Drawing for the job (mm, zero at the part's lowest x, y, z). A direction names the side the tool comes from. Coordinates: 2 decimals unless noted, no trailing zeros. Write each loop counter-clockwise with the first axis right and the second up, starting at its lowest first coordinate (ties: lowest second). Pieces come first, ordered by that corner, then holes. Notation, with made-up numbers: M 40.5,68.25 L 70.5,68.25 A10 cw 70.5,86.25 Z; hole C 5,58.5 d2. An arc over 180 degrees is marked long. Put each result on its own line as item: value. Start each with the question number.
Q1. Cut at A-A (z = 21.5). Write the cut outline in (x, y), then the cut area to 3 significant figures.
Q2. Drill centre lines: line 1 along X through (y, z) = (1.6, 21.25); line 2 along Z through (x, y) = (38.5, 2.2); line 3 along X through (y, z) = (1.25, 5.25). Where is each one in solid material? Low to high.
Q3. Which spindle directions (+Z, -Z, +X, -X, +Y, -Y) get a long thin tool onto all of the face, cutting with end or side? Do the marked faces 1, 2 and 3. Say none if no direction does.
Q4. Drop flat-ended pins along their axis: pin 1 (1.2 mm diameter, centred on y = 1.5, z = 5.5, fed in from +X); pin 2 (1.2 mm diameter, centred on y = 1, z = 3.5, fed in from -X); pin 3 (2 mm diameter, centred on x = 2.5, y = 2, fed in from -Z). Give the stop position or say it passes through.
Q5. Cut at C-C (x = 17). Write the cut outline in (y, z).
Q6. Cut at D-D (x = 38). Write the cut outline in (y, z).
Q7. Cut at B-B (y = 1.05). Write the cut outline in (x, z), then the cut area to 3 significant figures.
Q8. Pull direction X, two halves, no side cores. Call the marked faces 4, 5, 6 and 7: pulls with the +X half, pulls with the -X half, needs draft (parallel to the pull), parting line crosses it, or undercut.
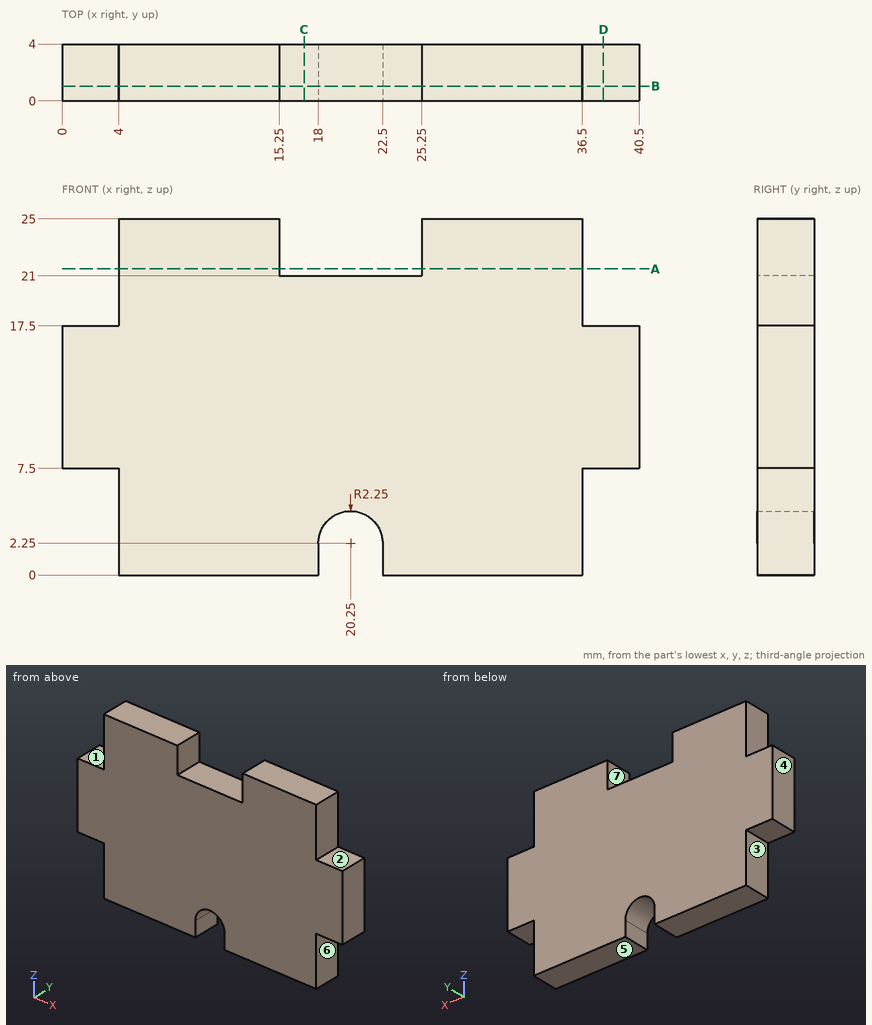
Computed values:
1. outline: M 4,0 L 15.25,0 L 15.25,4 L 4,4 Z; M 25.25,0 L 36.5,0 L 36.5,4 L 25.25,4 Z
1. area: 90.0 mm2
2. line 1: 4 to 15.25, 25.25 to 36.5
2. line 2: 7.5 to 17.5
2. line 3: 4 to 36.5
3. face 1: +Z, -X, +Y, -Y
3. face 2: +Z, +X, +Y, -Y
3. face 3: -Z, -X, +Y, -Y
4. pin 1: x = 36.5
4. pin 2: x = 4
4. pin 3: z = 7.5
5. outline: M 0,0 L 4,0 L 4,21 L 0,21 Z
6. outline: M 0,7.5 L 4,7.5 L 4,17.5 L 0,17.5 Z
7. outline: M 0,7.5 L 4,7.5 L 4,0 L 18,0 L 18,2.25 A2.25 cw 22.5,2.25 L 22.5,0 L 36.5,0 L 36.5,7.5 L 40.5,7.5 L 40.5,17.5 L 36.5,17.5 L 36.5,25 L 25.25,25 L 25.25,21 L 15.25,21 L 15.25,25 L 4,25 L 4,17.5 L 0,17.5 Z
7. area: 834 mm2
8. face 4: pulls with the -X half
8. face 5: needs draft
8. face 6: pulls with the +X half
8. face 7: undercut
